Autodesk Inventor part; units mm, degrees
ref_plane "YZ Plane" through (0, 0, 0) normal (1, 0, 0) x (0, 1, 0)
ref_plane "XZ Plane" through (0, 0, 0) normal (0, 1, 0) x (-1, 0, 0)
ref_plane "XY Plane" through (0, 0, 0) normal (0, 0, 1) x (1, 0, 0)
sketch "Skizze4" plane through (0, 0, 0) normal (0, 1, 0) x (-1, 0, 0)
  line L0 (-23.6102, 57) -> (23.6102, 57)
  line L1 (23.6102, 57) -> (57, 23.6102)
  line L2 (57, 23.6102) -> (57, -23.6102)
  line L3 (57, -23.6102) -> (23.6102, -57)
  line L4 (23.6102, -57) -> (-23.6102, -57)
  line L5 (-23.6102, -57) -> (-57, -23.6102)
  line L6 (-57, -23.6102) -> (-57, 23.6102)
  line L7 (-57, 23.6102) -> (-23.6102, 57)
  line L8 (0, -79.8) -> (0, 79.8) construction
  line L9 (79.8, 0) -> (-79.8, 0) construction
  circle A0 centre (0, 0) radius 40
  dimension "d4" = 114
  dimension "d5" = 80
extrude "Extrusion2" add sketch "Skizze4" along normal blind 2.5
sketch "Skizze5" plane through (0, 2.5, 0) normal (0, 1, 0) x (1, 0, 0)
  circle A0 centre (0, 0) radius 40
  line L0 (-23.6102, -57) -> (23.6102, -57)
  line L1 (23.6102, -57) -> (57, -23.6102)
  line L2 (57, -23.6102) -> (57, 23.6102)
  line L3 (57, 23.6102) -> (23.6102, 57)
  line L4 (23.6102, 57) -> (-23.6102, 57)
  line L5 (-23.6102, 57) -> (-57, 23.6102)
  line L6 (-57, 23.6102) -> (-57, -23.6102)
  line L7 (-57, -23.6102) -> (-23.6102, -57)
  line L8 (-52, 21.5391) -> (-21.5391, 52)
  line L9 (-21.5391, 52) -> (21.5391, 52)
  line L10 (21.5391, 52) -> (52, 21.5391)
  line L11 (52, 21.5391) -> (52, -21.5391)
  line L12 (52, -21.5391) -> (21.5391, -52)
  line L13 (21.5391, -52) -> (-21.5391, -52)
  line L14 (-21.5391, -52) -> (-52, -21.5391)
  line L15 (-52, -21.5391) -> (-52, 21.5391)
  dimension "d8" = 5
extrude "Extrusion3" add sketch "Skizze5" along normal blind 2.5 contours L8 L9 L10 L11 L12 L13 L14 L15
sketch "Skizze6" plane through (0, 5, 0) normal (0, 1, 0) x (1, 0, 0)
  circle A0 centre (0, 0) radius 40 construction
  line L0 (-21.5391, 52) -> (-52, 21.5391) construction
  line L1 (-52, 21.5391) -> (-52, -21.5391) construction
  line L2 (-52, -21.5391) -> (-21.5391, -52) construction
  line L3 (-21.5391, -52) -> (21.5391, -52) construction
  line L4 (21.5391, -52) -> (52, -21.5391) construction
  line L5 (52, -21.5391) -> (52, 21.5391) construction
  line L6 (52, 21.5391) -> (21.5391, 52) construction
  line L7 (21.5391, 52) -> (-21.5391, 52) construction
  line L8 (0, 79.8) -> (0, -79.8) construction
  point P0 (0, 48)
  point P1 (-48, 0)
  point P2 (0, -48)
  point P3 (48, 0)
  dimension "d11" = 48
  dimension "d14" = 360
hole "Bohrung1" at (0, 5, -48) at (-48, 5, 0) at (0, 5, 48) at (48, 5, 0) direction (0, -1, 0) diameter 4 end through all
sketch "Skizze7" plane through (0, 2.5, 0) normal (0, 1, 0) x (1, 0, 0)
  line L0 (-21.5391, 52) -> (21.5391, 52)
  line L1 (21.5391, 52) -> (52, 21.5391)
  line L2 (52, 21.5391) -> (52, -21.5391)
  line L3 (52, -21.5391) -> (21.5391, -52)
  line L4 (21.5391, -52) -> (-21.5391, -52)
  line L5 (-21.5391, -52) -> (-52, -21.5391)
  line L6 (-52, -21.5391) -> (-52, 21.5391)
  line L7 (-52, 21.5391) -> (-21.5391, 52)
  line L8 (-23.6102, -57) -> (23.6102, -57)
  line L9 (23.6102, -57) -> (57, -23.6102)
  line L10 (57, -23.6102) -> (57, 23.6102)
  line L11 (57, 23.6102) -> (23.6102, 57)
  line L12 (23.6102, 57) -> (-23.6102, 57)
  line L13 (-23.6102, 57) -> (-57, 23.6102)
  line L14 (-57, 23.6102) -> (-57, -23.6102)
  line L15 (-57, -23.6102) -> (-23.6102, -57)
  point P0 (0, 0)
extrude "Extrusion4" cut sketch "Skizze7" against normal blind 1
sketch "Skizze8" plane through (0, 0, 0) normal (0, -1, 0) x (1, 0, 0)
  circle A0 centre (0, 48) radius 2
  circle A1 centre (0, -48) radius 2
  circle A2 centre (-48, 0) radius 2
  circle A3 centre (48, 0) radius 2
  circle A4 centre (0, 0) radius 40
  line L0 (23.6102, 57) -> (-23.6102, 57)
  line L1 (-23.6102, 57) -> (-57, 23.6102)
  line L2 (-57, 23.6102) -> (-57, -23.6102)
  line L3 (-57, -23.6102) -> (-23.6102, -57)
  line L4 (-23.6102, -57) -> (23.6102, -57)
  line L5 (23.6102, -57) -> (57, -23.6102)
  line L6 (57, -23.6102) -> (57, 23.6102)
  line L7 (57, 23.6102) -> (23.6102, 57)
extrude "Extrusion5" add sketch "Skizze8" along normal blind 1
sketch "Skizze9" plane through (0, 5, 0) normal (0, 1, 0) x (1, 0, 0)
  circle A0 centre (0, -48) radius 2
  circle A1 centre (0, 48) radius 2
  circle A2 centre (-48, 0) radius 2
  circle A3 centre (48, 0) radius 2
  circle A4 centre (0, 0) radius 40
  line L0 (-21.5391, 52) -> (-52, 21.5391)
  line L1 (-52, 21.5391) -> (-52, -21.5391)
  line L2 (-52, -21.5391) -> (-21.5391, -52)
  line L3 (-21.5391, -52) -> (21.5391, -52)
  line L4 (21.5391, -52) -> (52, -21.5391)
  line L5 (52, -21.5391) -> (52, 21.5391)
  line L6 (52, 21.5391) -> (21.5391, 52)
  line L7 (21.5391, 52) -> (-21.5391, 52)
extrude "Extrusion6" cut sketch "Skizze9" against normal blind 0.5 contours A0 | A1 | A2 | A3 | L7 L6 L5 L4 L3 L2 L1 L0
sketch "Skizze10" plane through (0, 4.5, 0) normal (0, 1, 0) x (1, 0, 0)
  point P0 (0, 0)
sketch "Skizze11" plane through (0, 4.5, 0) normal (0, 1, 0) x (1, 0, 0)
  circle A0 centre (0, -48) radius 2
  circle A1 centre (0, 48) radius 2
  circle A2 centre (-48, 0) radius 2
  circle A3 centre (48, 0) radius 2
  circle A4 centre (0, 0) radius 40
  line L0 (-52, 21.5391) -> (-21.5391, 52)
  line L1 (-52, -21.5391) -> (-52, 21.5391)
  line L2 (-21.5391, -52) -> (-52, -21.5391)
  line L3 (21.5391, -52) -> (-21.5391, -52)
  line L4 (52, -21.5391) -> (21.5391, -52)
  line L5 (52, 21.5391) -> (52, -21.5391)
  line L6 (21.5391, 52) -> (52, 21.5391)
  line L7 (-21.5391, 52) -> (21.5391, 52)
extrude "Extrusion7" cut sketch "Skizze11" against normal blind 1
sketch "Skizze12" plane through (0, 1.5, 0) normal (0, 1, 0) x (1, 0, 0)
  line L0 (-21.5391, 52) -> (-52, 21.5391)
  line L1 (21.5391, 52) -> (-21.5391, 52)
  line L2 (52, 21.5391) -> (21.5391, 52)
  line L3 (52, -21.5391) -> (52, 21.5391)
  line L4 (21.5391, -52) -> (52, -21.5391)
  line L5 (-21.5391, -52) -> (21.5391, -52)
  line L6 (-52, -21.5391) -> (-21.5391, -52)
  line L7 (-52, 21.5391) -> (-52, -21.5391)
  line L8 (23.6102, -57) -> (-23.6102, -57)
  line L9 (57, -23.6102) -> (23.6102, -57)
  line L10 (57, 23.6102) -> (57, -23.6102)
  line L11 (23.6102, 57) -> (57, 23.6102)
  line L12 (-23.6102, 57) -> (23.6102, 57)
  line L13 (-57, 23.6102) -> (-23.6102, 57)
  line L14 (-57, -23.6102) -> (-57, 23.6102)
  line L15 (-23.6102, -57) -> (-57, -23.6102)
  point P0 (0, 0)
extrude "Extrusion8" cut sketch "Skizze12" against normal blind 1
properties part number "Stage3" material "3.3547 AlMg4,5Mn (AW-5083/H111)"
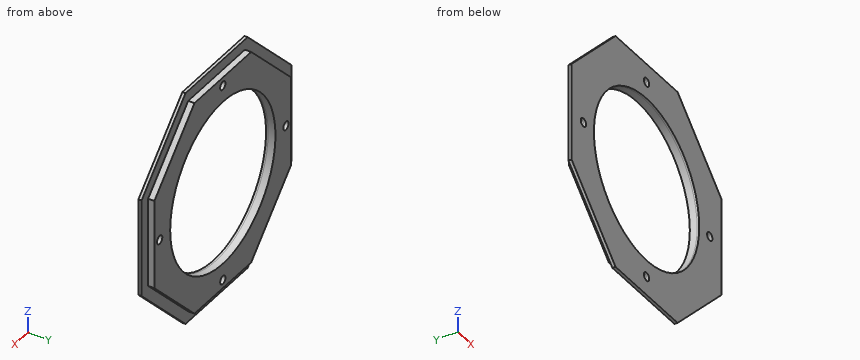
Work out the finished part from the listing and answer in its coordinate system (mm). Coordinates: 2 decimals unless noted, no trailing zeros. Loops run counter-clockwise (first coordinate to the right, second up) from the corner with the lowest first, then second, coordinate; pieces in that order, holes last. Notation, with made-up numbers: (12.5, -25) -> (41.5, -25) arc R31 ccw to (41.5, 12) -> close; hole circle Ø8 at (52.25, 3.5). An arc over 180 degrees is marked (long way). Write each question's results on one line, items separated by ' | '. Start each with the question number.
1) Consider line 1 along X through (y, z) = (2.15, 0); line 2 along X through (y, z) = (-0.25, 0). Determine where each line is inside the solid, lowest interval first.
2) Find section C-C on x = 48. Determine the outline of the cut face in (y, z).
3) Find section B-B on y = 1.2. Determine the outline of the cut face in (x, z), then the cut area to 3 significant figures.
4) Flat-ended cylindrical pins translate along their axes: P1, Ø3.5, axis at x = -48, z = 0, coming from the +Y side; P2, Ø2.5, axis at x = 2, y = 2.5, coming from the -Z side; P3, Ø1, axis at x = 8.5, y = 1.5, coming from the +Z side; P4, Ø2.5, axis at y = 2.5, z = 10, coming from the +X side. Find the tip coordinate at first contact, or state that the pin passes through.
5) Find section D-D on z = -48. Determine the outline of the cut face in (x, y), then the cut area to 3 significant figures.
Response values:
1) line 1: x = -52 to -50, -46 to -40, 40 to 46, 50 to 52 | line 2: x = -57 to -50, -46 to -40, 40 to 46, 50 to 57
2) outline: (-1, -32.61) -> (0.5, -32.61) -> (0.5, -25.54) -> (3.5, -25.54) -> (3.5, -2) -> (-1, -2) -> close; (-1, 2) -> (3.5, 2) -> (3.5, 25.54) -> (0.5, 25.54) -> (0.5, 32.61) -> (-1, 32.61) -> close
3) outline: (-52, -21.54) -> (-21.54, -52) -> (21.54, -52) -> (52, -21.54) -> (52, 21.54) -> (21.54, 52) -> (-21.54, 52) -> (-52, 21.54) -> close; hole circle Ø4 at (-48, 0); hole circle Ø80 at (0, 0); hole circle Ø4 at (0, -48); hole circle Ø4 at (0, 48); hole circle Ø4 at (48, 0) | area: 3,880 mm^2
4) P1: passes through | P2: stops at z = -52 | P3: stops at z = 52 | P4: stops at x = 52
5) outline: (-32.61, -1) -> (-2, -1) -> (-2, 3.5) -> (-25.54, 3.5) -> (-25.54, 0.5) -> (-32.61, 0.5) -> close; (2, -1) -> (32.61, -1) -> (32.61, 0.5) -> (25.54, 0.5) -> (25.54, 3.5) -> (2, 3.5) -> close | area: 233 mm^2
